from build123d import *

# Parameters (mm, degrees)
ESQUISSE1_W             = 12.5
ESQUISSE1_H             = 70
BOSS_EXTRU_1_DEPTH      = 10
BOSS_EXTRU_2_DEPTH      = 35
ENL_V_MAT_EXTRU_1_DEPTH = 40
CONG_3_R                = 2


with BuildPart() as part:
    # Esquisse1 → Boss.-Extru.1 (new body)
    with BuildSketch(Plane.XY):
        Rectangle(ESQUISSE1_W, ESQUISSE1_H)
    extrude(amount=BOSS_EXTRU_1_DEPTH)

    # Esquisse2 → Boss.-Extru.2 (add)
    with BuildSketch(Plane(origin=(0, 0, 0), x_dir=(-1, 0, 0), z_dir=(0, 0, -1))):
        Polygon((6.25, 0), (0, 6.25), (-6.25, 0), (0, -6.25), align=None)
    extrude(amount=-BOSS_EXTRU_2_DEPTH)

    # Esquisse3 → Enlèv. mat.-Extru.1 (cut)
    with BuildSketch(Plane(origin=(0, 0, 0), x_dir=(-1, 0, 0), z_dir=(0, 0, -1))):
        Polygon((-3.889087297, 0), (0, 3.889087297), (3.889087297, 0), (0, -3.889087297), align=None)
    extrude(amount=-ENL_V_MAT_EXTRU_1_DEPTH, mode=Mode.SUBTRACT)

    # Congé3
    cong_3_edges = [part.edges().sort_by_distance(p)[0] for p in [
        (0, -35, 10),
        (0, -35, 0),
        (0, 35, 0),
        (0, 35, 10),
    ]]
    fillet(cong_3_edges, radius=CONG_3_R)


solid = part.part
Work out the finished part from the listing and answer in its coordinate system (mm). A direction names the side the tool comes from. Give positions to 0.01 mm unless a question says otherwise; leave off trailing zeros. Loops run counter-clockwise (first coordinate to the right, second up) from the corner with the lowest first, then second, coordinate; pieces in that order, holes last. Notation, with made-up numbers: (6.25, 64) - (56.25, 64) arc R26 cw to (56.25, 87) - close; hole circle Ø1 at (-38, 80.5). An arc over 180 degrees is marked (long way). Answer in a Markdown table with one row per item. Add a question column.
Q1. A tool of negligible diameter and unlimited length cuts with its end or side. For faces 4 (the flat face through (1.97, 1.92, 17.26)), 5 (the flat face through (3.17, -3.08, 22.32)), 6 (the flat face through (4.3, 0.5, 0)), 7 (the flat face through (3.08, 3.17, 22.32)), 8 (the flat face through (-3.17, 3.08, 22.32)), from which of +Z, -Z, +X, -X, +Y, -Y can it reach the whole face along a straight path? Write none if from no direction.
Q2. The part is cut by section D-D (z = 31.5). Determine the outline of the cut face in (x, y), and give its area (3 significant figures).
Q3. Each of these flat-tipped pins is pushed along its axis until it touches: P1, Ø6, axis at x = -3, y = 8, coming from the +Z side; P2, Ø1.5, axis at x = 1, z = 22.5, coming from the -Y side; P3, Ø2, axis at y = 2, z = 25.5, coming from the +X side; P4, Ø10, axis at y = 4.5, z = 28, coming from the -X side. Where does it stop, or does it pass through?
Q4. The part is cut by section A-A (z = 7). Determine the outline of the cut face in (x, y).
Q5. The part is cut by section C-C (y = -5.5). Determine the outline of the cut face in (x, z), and give its area (4 significant figures).
Q6. Determine the mould class of faces 1 (the flat face through (-3.08, -3.17, 22.32)), 2 (the flat face through (0, -16, 10)), 3 (the flat face through (-1.92, 1.97, 17.26)) for opening direction X: released by +X, released by -X, zero draft, split by the parting line, or undercut.
Q7. The part is cut by section B-B (x = 1.25). Determine the outline of the cut face in (y, z), and give its area (3 significant figures).
Q8. Consider line 1 along Z through (x, y) = (-0.75, -6); line 2 along X through (y, z) = (-3, 7.5); line 3 along Y through (x, z) = (3.25, 9). Determine where each line is inside the solid, lowest interval first.
Solution:
| question | item | result |
|---|---|---|
| 1 | face 4 | +Z, -Z |
| 1 | face 5 | +Z, +X, -Y |
| 1 | face 6 | -Z, +X, -X, +Y, -Y |
| 1 | face 7 | +Z, +X, +Y |
| 1 | face 8 | +Z, -X, +Y |
| 2 | outline | (-6.25, 0) - (0, -6.25) - (6.25, 0) - (0, 6.25) - close; hole (-3.89, 0) - (0, -3.89) - (3.89, 0) - (0, 3.89) - close |
| 2 | area | 47.9 mm² |
| 3 | P1 | stops at z = 10 |
| 3 | P2 | stops at y = -6 |
| 3 | P3 | stops at x = 5.25 |
| 3 | P4 | stops at x = -6.25 |
| 4 | outline | (-6.25, -35) - (6.25, -35) - (6.25, 35) - (-6.25, 35) - close; hole (-3.89, 0) - (0, -3.89) - (3.89, 0) - (0, 3.89) - close |
| 5 | outline | (-6.25, 0) - (6.25, 0) - (6.25, 10) - (0.75, 10) - (0.75, 35) - (-0.75, 35) - (-0.75, 10) - (-6.25, 10) - close |
| 5 | area | 162.5 mm² |
| 6 | face 1 | released by -X |
| 6 | face 2 | zero draft |
| 6 | face 3 | undercut |
| 7 | outline | (-35, 2) arc R2 ccw to (-33, 0) - (-2.64, 0) - (-2.64, 35) - (-5, 35) - (-5, 10) - (-33, 10) arc R2 ccw to (-35, 8) - close; (2.64, 0) - (33, 0) arc R2 ccw to (35, 2) - (35, 8) arc R2 ccw to (33, 10) - (5, 10) - (5, 35) - (2.64, 35) - close |
| 7 | area | 762 mm² |
| 8 | line 1 | z = 0 to 10 |
| 8 | line 2 | x = -6.25 to -0.89, 0.89 to 6.25 |
| 8 | line 3 | y = -34.73 to -0.64, 0.64 to 34.73 |
